Verification items for this drawing (mm, ordinates from the low corner). Round coordinates to 2 decimals unless told otherwise and drop trailing zeros. Order: outer loops, then holes, each group sorted by start corner. A loop starts at its lowest first (then second) coordinate and runs counter-clockwise, first axis right, second up. Notation, with made-up numbers: (24, 79.25) -> (45, 79.25) arc R15 cw to (45, 103.25) -> close; hole circle Ø6 at (-36, 63.5). An arc over 180 degrees is marked (long way). Answer in a Markdown table with one row per item. Add a question column.
1. Material ranges on L1, parallel to Y at x = 44.5, z = 46 (1 decimal); L2, parallel to X at y = 83.5, z = 4; L3, parallel to Y at x = 23, z = 15.5 (1 decimal), recorded low to high. Write a range as from..to.
2. Sectioned sample at A-A, the plane z = 78. Record the boundary of the cut face in (x, y) (1 decimal).
3. Sectioned sample at C-C, the plane x = 11.5. Record the boundary of the cut face in (y, z), then the cut area to 4 significant figures.
4. Sectioned sample at B-B, the plane y = 82.5. Record the boundary of the cut face in (x, z), then the cut area to 3 significant figures.
5. Depth check by flat-ended pin: P1, Ø6, axis at x = 37, z = 26, coming from the +Y side. Enter the tip coordinate at first touch or a pass-through.
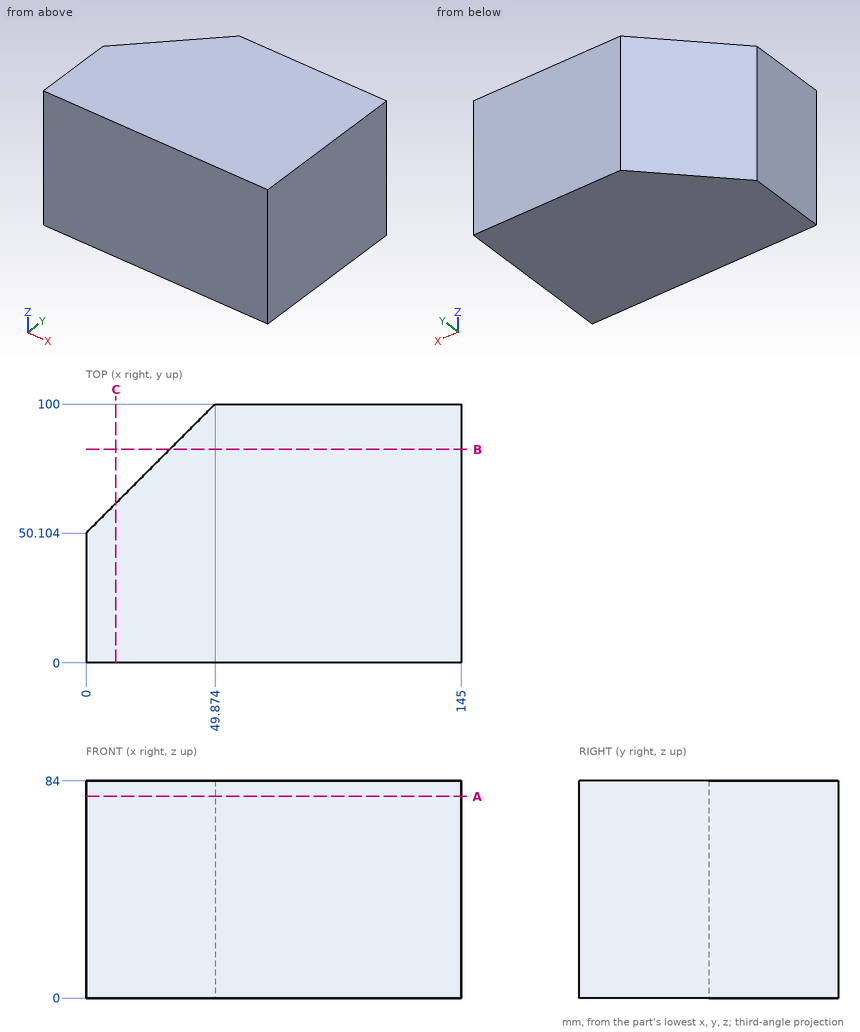
Answer key:
| question | item | result |
|---|---|---|
| 1 | L1 | y = 0..94.6 |
| 1 | L2 | x = 33.38..145 |
| 1 | L3 | y = 0..73.1 |
| 2 | outline | (0, 0) -> (145, 0) -> (145, 100) -> (49.9, 100) -> (0, 50.1) -> close |
| 3 | outline | (0, 0) -> (61.61, 0) -> (61.61, 84) -> (0, 84) -> close |
| 3 | area | 5,175 mm² |
| 4 | outline | (32.38, 0) -> (145, 0) -> (145, 84) -> (32.38, 84) -> close |
| 4 | area | 9,460 mm² |
| 5 | P1 | stops at y = 90.12 |
